```python
from build123d import *

# Parameters (mm, degrees)
BOSS_EXTRUDE1_DEPTH = 1.5748
SKETCH2_R           = 0.508
SKETCH2_R_2         = 0.762
CUT_EXTRUDE1_DEPTH  = 104.686284508


with BuildPart() as part:
    # Sketch1 → Boss-Extrude1 (new body)
    with BuildSketch(Plane.XY):
        Polygon((0, 49.9872), (1.27, 51.2572), (30.9372, 51.2572), (33.02, 53.34), (86.36, 53.34), (88.9, 50.8), (88.9, 2.54), (86.36, 0), (33.02, 0), (30.48, 2.54), (0.635, 2.54), (0, 3.175), align=None)
    extrude(amount=BOSS_EXTRUDE1_DEPTH)

    # Sketch2 → Cut-Extrude1 (cut, through all)
    with BuildSketch(Plane.XY.offset(1.5748)):
        with Locations((3.429, 8.636)):
            Circle(SKETCH2_R)
        with Locations((3.429, 11.176)):
            Circle(SKETCH2_R)
        with Locations((3.429, 13.716)):
            Circle(SKETCH2_R)
        with Locations((3.429, 16.256)):
            Circle(SKETCH2_R)
        with Locations((5.08, 25.4)):
            Circle(SKETCH2_R_2)
        with Locations((5.08, 30.48)):
            Circle(SKETCH2_R_2)
        with Locations((5.08, 35.56)):
            Circle(SKETCH2_R_2)
        with Locations((5.08, 40.64)):
            Circle(SKETCH2_R_2)
        with Locations((85.4456, 4.4958)):
            Circle(SKETCH2_R)
        with Locations((85.4456, 7.0358)):
            Circle(SKETCH2_R)
        with Locations((85.4456, 9.5758)):
            Circle(SKETCH2_R)
        with Locations((85.4456, 12.1158)):
            Circle(SKETCH2_R)
        with Locations((85.4456, 14.6558)):
            Circle(SKETCH2_R)
        with Locations((85.4456, 17.1958)):
            Circle(SKETCH2_R)
        with Locations((85.4456, 19.7358)):
            Circle(SKETCH2_R)
        with Locations((85.4456, 22.2758)):
            Circle(SKETCH2_R)
        with Locations((34.4932, 50.8)):
            Circle(SKETCH2_R)
        with Locations((37.0332, 50.8)):
            Circle(SKETCH2_R)
        with Locations((39.5732, 50.8)):
            Circle(SKETCH2_R)
        with Locations((42.1132, 50.8)):
            Circle(SKETCH2_R)
        with Locations((44.6532, 50.8)):
            Circle(SKETCH2_R)
        with Locations((47.1932, 50.8)):
            Circle(SKETCH2_R)
        with Locations((52.2732, 50.8)):
            Circle(SKETCH2_R)
        with Locations((54.8132, 50.8)):
            Circle(SKETCH2_R)
        with Locations((57.3532, 50.8)):
            Circle(SKETCH2_R)
        with Locations((59.8932, 50.8)):
            Circle(SKETCH2_R)
        with Locations((62.4332, 50.8)):
            Circle(SKETCH2_R)
        with Locations((64.9732, 50.8)):
            Circle(SKETCH2_R)
        with Locations((67.5132, 50.8)):
            Circle(SKETCH2_R)
        with Locations((70.0532, 50.8)):
            Circle(SKETCH2_R)
        with Locations((34.4932, 2.54)):
            Circle(SKETCH2_R)
        with Locations((37.0332, 2.54)):
            Circle(SKETCH2_R)
        with Locations((39.5732, 2.54)):
            Circle(SKETCH2_R)
        with Locations((42.1132, 2.54)):
            Circle(SKETCH2_R)
        with Locations((44.6532, 2.54)):
            Circle(SKETCH2_R)
        with Locations((47.1932, 2.54)):
            Circle(SKETCH2_R)
        with Locations((49.7332, 2.54)):
            Circle(SKETCH2_R)
        with Locations((52.2732, 2.54)):
            Circle(SKETCH2_R)
        with Locations((56.0832, 2.54)):
            Circle(SKETCH2_R)
        with Locations((58.6232, 2.54)):
            Circle(SKETCH2_R)
        with Locations((61.1632, 2.54)):
            Circle(SKETCH2_R)
        with Locations((63.7032, 2.54)):
            Circle(SKETCH2_R)
        with Locations((66.2432, 2.54)):
            Circle(SKETCH2_R)
        with Locations((68.7832, 2.54)):
            Circle(SKETCH2_R)
        with Locations((71.3232, 2.54)):
            Circle(SKETCH2_R)
        with Locations((73.8632, 2.54)):
            Circle(SKETCH2_R)
        with Locations((76.4032, 2.54)):
            Circle(SKETCH2_R)
        with Locations((78.9432, 2.54)):
            Circle(SKETCH2_R)
    extrude(amount=-CUT_EXTRUDE1_DEPTH, mode=Mode.SUBTRACT)


solid = part.part
```
Could you check a few things on this model? Use its own coordinates, in mm. A direction names the side the tool comes from. Give positions to 0.01 mm unless a question says otherwise; leave off trailing zeros. Use one line per item in the form item = value.
1. I need wall thicknesses on probe 1 along Y at (x, z) = (5.5, 0.35); probe 2 along Y at (x, z) = (74, 0.35); probe 3 along X at (y, z) = (4.5, 0.35). Which ranges of each line are inside material? Lowest first, please.
Response values:
probe_1 = 2.54 to 24.76, 26.04 to 29.84, 31.12 to 34.92, 36.2 to 40, 41.28 to 51.26
probe_2 = 0 to 2.05, 3.03 to 53.34
probe_3 = 0 to 84.94, 85.95 to 88.9
2. On a 3-axis mill with a long thin cutter (end or side, diameter ignored), from which of +Z, -Z, +X, -X, +Y, -Y can I reach the whole of each face in a straight line? I mean faces 1 (the face through (87.65, 1.29, 0.78)), 2 (the face through (16, 51.257, 1)), 3 (the face through (16, 2.54, 1)). Say none if no direction works.
Response values:
face_1 = +Z, -Z, +X, -Y
face_2 = +Z, -Z, -X, +Y
face_3 = +Z, -Z, -X, -Y
3. I want a section at A-A (z = 1.2). Give the number of separate pieces and of enclosed holes in the cut face, and give its area (3 significant figures).
Response values:
separate_pieces = 1
enclosed_holes = 48
area = 4,540 mm²
